The drawing under review shows one solid part. Ordinate dimensions are in mm from its lowest x, y, z. Give positions to 0.01 mm unless a question says otherwise; leave off trailing zeros. Order: outer loops, then holes, each group sorted by start corner. A loop starts at its lowest first (then second) coordinate and runs counter-clockwise, first axis right, second up. Notation, with made-up numbers: (-4.75, 32) - (50.25, 32) arc R16 cw to (50.25, 43) - close; hole circle Ø8 at (8, 54). An arc over 180 degrees is marked (long way). Use CSV: the item, a comma, the result in double quotes.
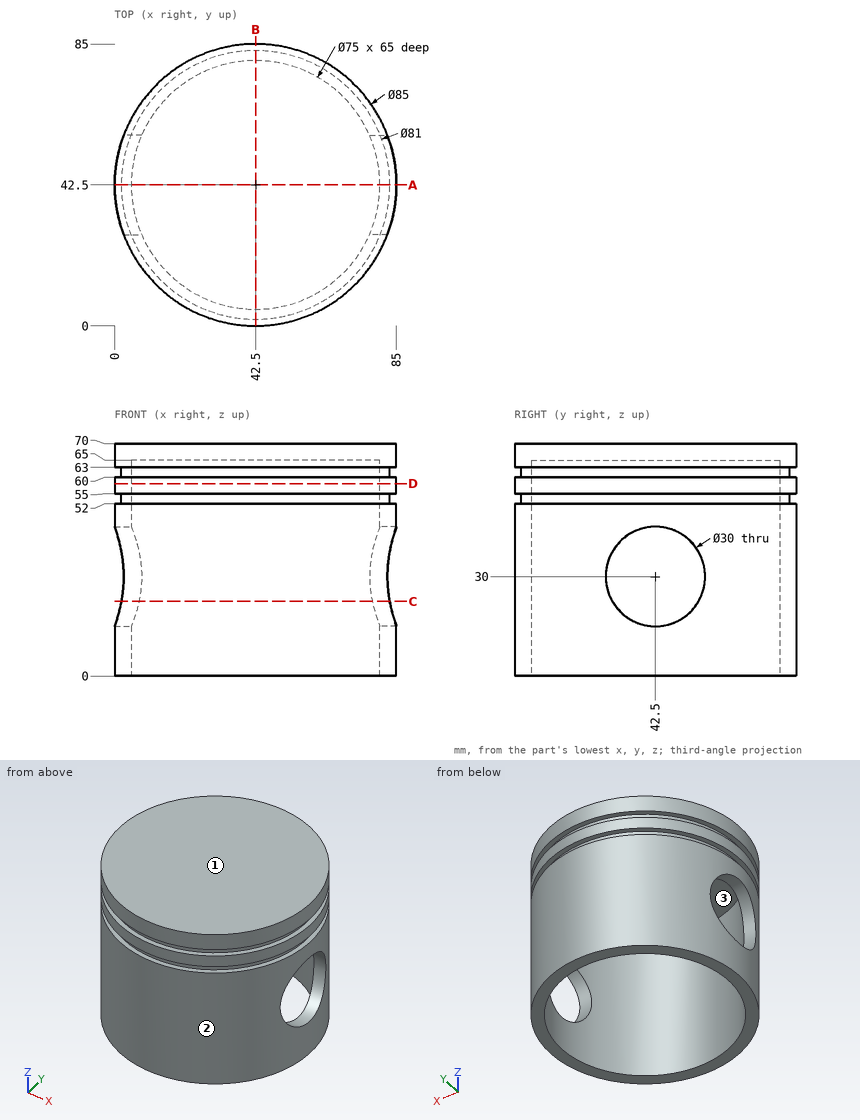
Item 1: Mouldability with a two-part tool opening along Y and no side actions: class the marked faces 1, 2 and 3 as pulls with the +Y half, pulls with the -Y half, needs draft (parallel to the pull), parting line crosses it, or undercut.
Results list:
face 1,"needs draft"
face 2,"parting line crosses it"
face 3,"undercut"
Item 2: Clearance check with flat-ended pins moving along their axes: pin 1 (1.5 mm diameter, centred on y = 10, z = 13.5, fed in from -X); pin 2 (4 mm diameter, centred on y = 20.5, z = 62, fed in from -X); pin 3 (3 mm diameter, centred on x = 40.5, z = 55.5, fed in from +Y); pin 4 (18 mm diameter, centred on y = 42.5, z = 30, fed in from +X). State where each tip first meets the part, or that it passes through.
Results list:
pin 1,"stops at x = 14.25"
pin 2,"stops at x = 5.14"
pin 3,"stops at y = 85"
pin 4,"passes through"
Item 3: Take a section at A-A, the plane y = 42.5. State how many separate pieces and enclosed holes the cut face has, and give its area (3 significant figures).
Results list:
separate pieces,"3"
enclosed holes,"0"
area,"751 mm2"
Item 4: Wall thickness on L1, parallel to Z at x = 65, y = 78; L2, parallel to Y at x = 42.5, z = 37; L3, parallel to Z at x = 68, y = 42: over which ranges is each line inside the solid? List them lowest first.
Results list:
L1,"z = 0 to 52, 55 to 60, 63 to 70"
L2,"y = 0 to 5, 80 to 85"
L3,"z = 65 to 70"
Item 5: Take a section at B-B, the plane x = 42.5. Give the boundary of the cut face in (y, z), and give its area (3 significant figures).
Results list:
outline,"(0, 0) - (5, 0) - (5, 65) - (80, 65) - (80, 0) - (85, 0) - (85, 52) - (83, 52) - (83, 55) - (85, 55) - (85, 60) - (83, 60) - (83, 63) - (85, 63) - (85, 70) - (0, 70) - (0, 63) - (2, 63) - (2, 60) - (0, 60) - (0, 55) - (2, 55) - (2, 52) - (0, 52) - close"
area,"1,050 mm2"
Item 6: Take a section at C-C, the plane z = 22.5. Give the boundary of the cut face in (x, y), and give its area (3 significant figures).
Results list:
outline,"(2.03, 29.51) arc R42.5 ccw to (82.97, 29.51) - (77.68, 29.51) arc R37.5 cw to (7.32, 29.51) - close; (2.03, 55.49) - (7.32, 55.49) arc R37.5 cw to (77.68, 55.49) - (82.97, 55.49) arc R42.5 ccw to start"
area,"992 mm2"
Item 7: Take a section at D-D, the plane z = 58. Give the boundary of the cut face in (x, y), and give its area (3 significant figures).
Results list:
outline,"circle Ø85 at (42.5, 42.5); hole circle Ø75 at (42.5, 42.5)"
area,"1,260 mm2"
